```python
from build123d import *

# Parameters (mm, degrees)
SKETCH2_W           = 28.75
SKETCH2_H           = 28.75
BOSS_EXTRUDE1_DEPTH = 5
CHAMFER1_SIZE       = 2.5
SKETCH3_R           = 1.25
CUT_EXTRUDE1_DEPTH  = 1.25
SKETCH6_R           = 2.5
CUT_EXTRUDE2_DEPTH  = 3.75


with BuildPart() as part:
    # Sketch2 → Boss-Extrude1 (new body)
    with BuildSketch(Plane(origin=(0, 0, 0), x_dir=(1, 0, 0), z_dir=(0, 1, 0))):
        Rectangle(SKETCH2_W, SKETCH2_H)
    extrude(amount=BOSS_EXTRUDE1_DEPTH)

    # Chamfer1
    chamfer1_edges = [part.edges().sort_by_distance(p)[0] for p in [
        (-14.375, 5, 0),
        (0, 5, 14.375),
        (14.375, 5, 0),
        (0, 5, -14.375),
    ]]
    chamfer(chamfer1_edges, length=CHAMFER1_SIZE)

    # Sketch3 → Cut-Extrude1 (cut)
    with BuildSketch(Plane(origin=(0, 5, 0), x_dir=(1, 0, 0), z_dir=(0, 1, 0))):
        Circle(SKETCH3_R)
    extrude(amount=-CUT_EXTRUDE1_DEPTH, mode=Mode.SUBTRACT)

    # Sketch6 → Cut-Extrude2 (cut)
    with BuildSketch(Plane(origin=(0, 3.75, 0), x_dir=(1, 0, 0), z_dir=(0, 1, 0))):
        Circle(SKETCH6_R)
    extrude(amount=-CUT_EXTRUDE2_DEPTH, mode=Mode.SUBTRACT)


solid = part.part
```
Here's how the part is built. I have some questions about the finished solid (model axes, mm). A direction names the side the tool comes from. Give positions to 0.01 mm unless a question says otherwise; leave off trailing zeros. Write each loop counter-clockwise with the first axis right and the second up, starting at its lowest first coordinate (ties: lowest second). Pieces come first, ordered by that corner, then holes.
(1) Imagine slicing it at C-C, the plane y = 1.4. Write out the boundary of the cut face in (x, z) (3 decimals), and give its area (3 significant figures).
Output values:
outline: (-14.375, -14.375) - (14.375, -14.375) - (14.375, 14.375) - (-14.375, 14.375) - close; hole circle Ø5 at (0, 0)
area: 807 mm2
(2) Thinking about a two-plate mould opening in Z: for faces 3 (the face through (14.375, 1, 0)), 4 (the face through (0, 1, 14.375)), 5 (the face through (-0.54, 1.9, 2.44)), which applies, pulls with the +Z half, pulls with the -Z half, needs draft (parallel to the pull), parting line crosses it, or undercut?
Output values:
face 3: needs draft
face 4: pulls with the +Z half
face 5: undercut
(3) On a 3-axis mill with a long thin cutter (end or side, diameter ignored), from which of +Z, -Z, +X, -X, +Y, -Y can I reach the whole of each face in a straight line? I mean faces 1 (the face through (-13.108, 3.767, 0.201)), 2 (the face through (-1, 3.75, 1)). Say none if no direction works.
Output values:
face 1: +Z, -Z, -X, +Y
face 2: -Y
(4) Imagine slicing it at D-D, the plane x = -11.5. Write out the boundary of the cut face in (y, z) (3 decimals), and give its area (4 significant figures).
Output values:
outline: (0, -14.375) - (2.5, -14.375) - (5, -11.875) - (5, 11.875) - (2.5, 14.375) - (0, 14.375) - close
area: 137.5 mm2
(5) Imagine slicing it at A-A, the plane z = 0. Write out the boundary of the cut face in (x, y) (3 decimals).
Output values:
outline: (-14.375, 0) - (-2.5, 0) - (-2.5, 3.75) - (-1.25, 3.75) - (-1.25, 5) - (-11.875, 5) - (-14.375, 2.5) - close; (1.25, 3.75) - (2.5, 3.75) - (2.5, 0) - (14.375, 0) - (14.375, 2.5) - (11.875, 5) - (1.25, 5) - close
(6) If I drill on L1, parallel to Z at x = 0, y = 1.2 (3 decimals); L2, parallel to Y at x = -2, z = -1, over which ranges is the centre line in solid material (lowest first)?
Output values:
L1: z = -14.375 to -2.5, 2.5 to 14.375
L2: y = 3.75 to 5
(7) Imagine slicing it at B-B, the plane x = 0. Write out the boundary of the cut face in (y, z) (3 decimals), and give its area (3 significant figures).
Output values:
outline: (0, -14.375) - (2.5, -14.375) - (5, -11.875) - (5, -1.25) - (3.75, -1.25) - (3.75, -2.5) - (0, -2.5) - close; (0, 2.5) - (3.75, 2.5) - (3.75, 1.25) - (5, 1.25) - (5, 11.875) - (2.5, 14.375) - (0, 14.375) - close
area: 116 mm2
